Check sheet for the drawn part. Datum: minimum x, y, z corner. Units: mm. A direction names the side the tool comes from. Round coordinates to 2 decimals unless told otherwise and drop trailing zeros. Loops run counter-clockwise (first coordinate to the right, second up) from the corner with the lowest first, then second, coordinate; pieces in that order, holes last.
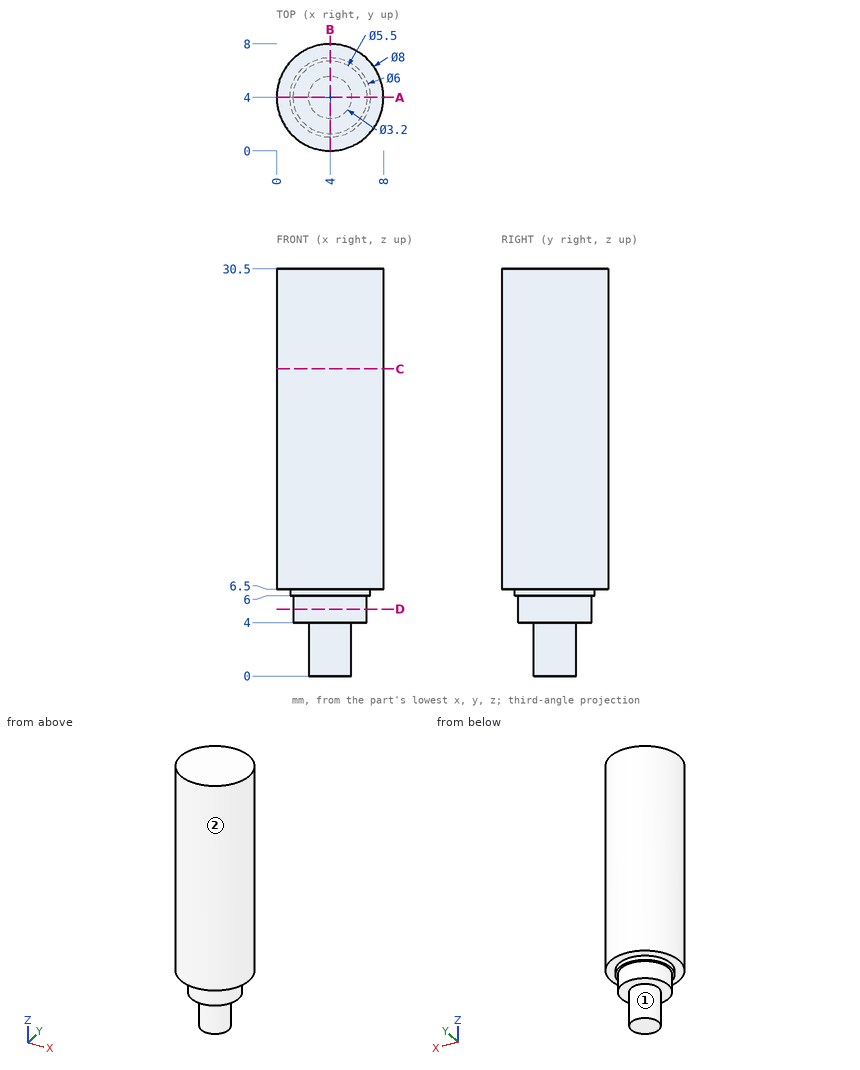
1) Access from +Z, -Z, +X, -X, +Y, -Y to the whole of each face (thin tool, end or side, straight path). Record for the marked faces 1 and 2.
Report:
face 1: -Z
face 2: +Z, -Z
2) Sectioned sample at D-D, the plane z = 5. Record the cut outline in (x, y).
Report:
outline: circle Ø5.5 at (4, 4)
3) Scan lines: line 1 along Z through (x, y) = (4.75, 5.5); line 2 along Z through (x, y) = (7.5, 5.75); line 3 along Y through (x, z) = (5, 22). Record each from-to range of solid material in increasing order.
Report:
line 1: z = 4 to 30.5
line 2: z = 6.5 to 30.5
line 3: y = 0.13 to 7.87
4) Gauge pin test, flat ends, axial feed: pin 1 (1 mm diameter, centred on y = 5, z = 4, fed in from +X); pin 2 (1.6 mm diameter, centred on x = 5, y = 3, fed in from -Z); pin 3 (1 mm diameter, centred on y = 2.5, z = 23.5, fed in from +X); pin 4 (1 mm diameter, centred on y = 3, z = 26, fed in from -X). Record the tip position at first contact, or that the pin passes through.
Report:
pin 1: stops at x = 6.7
pin 2: stops at z = 0
pin 3: stops at x = 7.87
pin 4: stops at x = 0.03
5) Sectioned sample at C-C, the plane z = 23. Record the cut outline in (x, y), then the cut area to 3 significant figures.
Report:
outline: circle Ø8 at (4, 4)
area: 50.3 mm2
6) Sectioned sample at A-A, the plane y = 4. Record the cut outline in (x, z), then the cut area to 3 significant figures.
Report:
outline: (0, 6.5) - (1, 6.5) - (1, 6) - (1.25, 6) - (1.25, 4) - (2.4, 4) - (2.4, 0) - (5.6, 0) - (5.6, 4) - (6.75, 4) - (6.75, 6) - (7, 6) - (7, 6.5) - (8, 6.5) - (8, 30.5) - (0, 30.5) - close
area: 219 mm2
